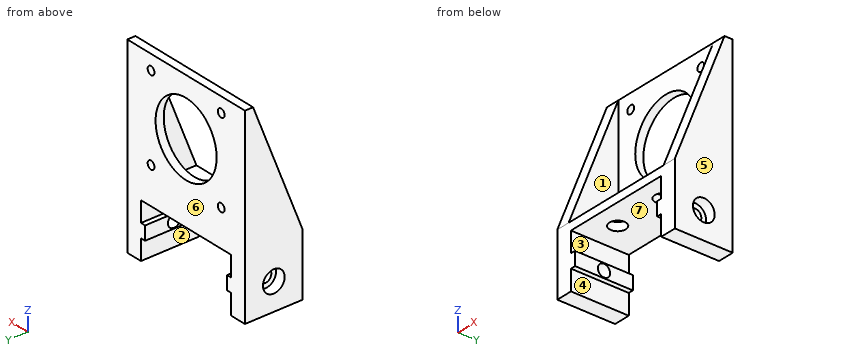
from build123d import *

# Parameters (mm, degrees)
SKETCH1_W           = 42
SKETCH1_H           = 21.3
BOSS_EXTRUDE1_DEPTH = 3
SKETCH2_R           = 3
CUT_EXTRUDE1_DEPTH  = 3
SKETCH4_W           = 42
SKETCH4_H           = 50
SKETCH4_R           = 1.5
SKETCH4_R_2         = 13.5
BOSS_EXTRUDE2_DEPTH = 3
BOSS_EXTRUDE3_DEPTH = 5
BOSS_EXTRUDE4_START = -42
BOSS_EXTRUDE4_DEPTH = 5
SKETCH6_W           = 6.04
SKETCH6_H           = 19.96
BOSS_EXTRUDE5_DEPTH = 21.3
SKETCH8_W           = 1.829995551
SKETCH8_H           = 5.02
BOSS_EXTRUDE6_DEPTH = 21.3
SKETCH7_R           = 2.25
CUT_EXTRUDE2_DEPTH  = 10
SKETCH9_R           = 4
CUT_EXTRUDE3_DEPTH  = 3.8


with BuildPart() as part:
    # Sketch1 → Boss-Extrude1 (new body)
    with BuildSketch(Plane.XY):
        with Locations((98.144783915, 168.215968794)):
            Rectangle(SKETCH1_W, SKETCH1_H)
    extrude(amount=BOSS_EXTRUDE1_DEPTH)

    # Sketch2 → Cut-Extrude1 (cut)
    with BuildSketch(Plane.XY.offset(3)):
        with Locations((108.644783915, 166.065968794)):
            Circle(SKETCH2_R)
        with Locations((88.644783915, 166.065968794)):
            Circle(SKETCH2_R)
    extrude(amount=-CUT_EXTRUDE1_DEPTH, mode=Mode.SUBTRACT)

    # Sketch4 → Boss-Extrude2 (add)
    with BuildSketch(Plane(origin=(0, 178.865968794, 0), x_dir=(-1, 0, 0), z_dir=(0, 1, 0))):
        with Locations((-98.144783915, 25)):
            Rectangle(SKETCH4_W, SKETCH4_H)
        with Locations((-113.644783915, 44.500179206)):
            Circle(SKETCH4_R, mode=Mode.SUBTRACT)
        with Locations((-82.644783915, 44.500179206)):
            Circle(SKETCH4_R, mode=Mode.SUBTRACT)
        with Locations((-82.644783915, 13.500179206)):
            Circle(SKETCH4_R, mode=Mode.SUBTRACT)
        with Locations((-113.644783915, 13.500179206)):
            Circle(SKETCH4_R, mode=Mode.SUBTRACT)
        with Locations((-98.144783915, 29.000179206)):
            Circle(SKETCH4_R_2, mode=Mode.SUBTRACT)
    extrude(amount=-BOSS_EXTRUDE2_DEPTH)

    # Sketch5 → Boss-Extrude3 (add)
    with BuildSketch(Plane(origin=(119.144783915, 0, 0), x_dir=(0, 0, -1), z_dir=(1, 0, 0))):
        Polygon((0, 157.565968794), (0, 178.865968794), (-50, 178.865968794), (-50, 175.865968794), (-3, 157.565968794), align=None)
    extrude(amount=BOSS_EXTRUDE3_DEPTH)

    # Sketch5<3> → Boss-Extrude4 (add)
    with BuildSketch(Plane(origin=(119.144783915, 0, 0), x_dir=(0, 0, -1), z_dir=(1, 0, 0)).offset(BOSS_EXTRUDE4_START)):
        Polygon((0, 157.565968794), (0, 178.865968794), (-50, 178.865968794), (-50, 175.865968794), (-3, 157.565968794), align=None)
    extrude(amount=-BOSS_EXTRUDE4_DEPTH)

    # Sketch6 → Boss-Extrude5 (add)
    with BuildSketch(Plane(origin=(0, 178.865968794, 0), x_dir=(1, 0, 0), z_dir=(0, 1, 0))):
        with Locations((75.164783915, 9.98)):
            Rectangle(SKETCH6_W, SKETCH6_H)
    boss_extrude5 = extrude(amount=-BOSS_EXTRUDE5_DEPTH)

    # Sketch8 → Boss-Extrude6 (add)
    with BuildSketch(Plane(origin=(0, 157.565968794, 0), x_dir=(-1, 0, 0), z_dir=(0, -1, 0))):
        with Locations((-79.099781691, 9.98)):
            Rectangle(SKETCH8_W, SKETCH8_H)
    boss_extrude6 = extrude(amount=-BOSS_EXTRUDE6_DEPTH)

    # Sketch7 → Cut-Extrude2 (cut)
    with BuildSketch(Plane.ZY.offset(-72.144783915)):
        with Locations((-9.98, 168.215968794)):
            Circle(SKETCH7_R)
    cut_extrude2 = extrude(amount=-CUT_EXTRUDE2_DEPTH, mode=Mode.SUBTRACT)

    # Sketch9 → Cut-Extrude3 (cut)
    with BuildSketch(Plane.ZY.offset(-72.144783915)):
        with Locations((-9.98, 168.215968794)):
            Circle(SKETCH9_R)
    cut_extrude3 = extrude(amount=-CUT_EXTRUDE3_DEPTH, mode=Mode.SUBTRACT)

    # Mirror1: Boss-Extrude5, Boss-Extrude6, Cut-Extrude2, Cut-Extrude3 across plane
    add(boss_extrude5.mirror(Plane.ZY.offset(-98.144783915)))
    add(boss_extrude6.mirror(Plane.ZY.offset(-98.144783915)))
    add(cut_extrude2.mirror(Plane.ZY.offset(-98.144783915)), mode=Mode.SUBTRACT)
    add(cut_extrude3.mirror(Plane.ZY.offset(-98.144783915)), mode=Mode.SUBTRACT)


solid = part.part
Can you work these out from the model? Positions are in its coordinate system, mm. Face numbers are marked on the shaded views. A direction names the side the tool comes from. Coordinates: 2 decimals unless noted, no trailing zeros. Loops run counter-clockwise (first coordinate to the right, second up) from the corner with the lowest first, then second, coordinate; pieces in that order, holes last. Notation, with made-up numbers: (24, 25) - (53, 25) arc R15 cw to (53, 32) - close; hole circle Ø7 at (-27, -23). An arc over 180 degrees is marked (long way). Put each result on its own line as item: value. Start each with the question number.
Item 1: Suppose I cut it at B-B (x = 95). Please give me the cut outline in (y, z).
Item 2: Suppose I cut it at D-D (z = -10.5). Please give me the cut outline in (x, y).
Item 3: Which directions (+Z, -Z, +X, -X, +Y, -Y) give clear straight access to the entire face, cutting with the end or side of a thin tool? Please do the marked faces 1, 2 and 3.
Item 4: For pin 1 (5 mm diameter, centred on x = 110, y = 169.5, fed in from -Z); pin 2 (1.5 mm diameter, centred on x = 79, y = 168.5, fed in from +Z); pin 3 (4 mm diameter, centred on x = 113.64, z = 44.5, fed in from -Y), each with a flat end and sliding along its axis, tell me the tip position at first contact or that it passes through.
Item 5: If we mould it in two halves opening along X, with no side actions, what happens to the marked faces 4, 5, 6 and 7? For each: +X half, -X half, draft (parallel to the pull), parting line (faces both ways), or undercut.
Item 6: Suppose I cut it at A-A (z = -3.5). Please give me the cut outline in (x, y).
Item 7: Suppose I cut it at C-C (y = 177.5). Please give me the cut outline in (x, z), and give its area (3 significant figures).
Item 8: If I drill on line 1 along X through (y, z) = (169.5, -4); line 2 along X through (y, z) = (173.75, 17); line 3 along Z through (x, y) = (118, 176.75), over which ranges is the centre line in solid material (lowest first)?
Here are the results:
1. outline: (157.57, 0) - (178.87, 0) - (178.87, 15.87) - (175.87, 15.87) - (175.87, 3) - (157.57, 3) - close; (175.87, 42.13) - (178.87, 42.13) - (178.87, 50) - (175.87, 50) - close
2. outline: (72.14, 157.57) - (80.01, 157.57) - (80.01, 166.03) - (75.94, 166.03) - (75.94, 164.25) - (72.14, 164.25) - close; (72.14, 172.18) - (75.94, 172.18) - (75.94, 170.41) - (80.01, 170.41) - (80.01, 178.87) - (72.14, 178.87) - close; (116.27, 157.57) - (124.14, 157.57) - (124.14, 164.25) - (120.34, 164.25) - (120.34, 166.03) - (116.27, 166.03) - close; (116.27, 170.41) - (120.34, 170.41) - (120.34, 172.18) - (124.14, 172.18) - (124.14, 178.87) - (116.27, 178.87) - close
3. face 1: +Z, -Y
3. face 2: -Z, +Y, -Y
3. face 3: +Y, -Y
4. pin 1: z = 0
4. pin 2: z = 3
4. pin 3: y = 175.87
5. face 4: undercut
5. face 5: +X half
5. face 6: draft
5. face 7: undercut
6. outline: (72.14, 157.57) - (78.18, 157.57) - (78.18, 178.87) - (72.14, 178.87) - close; (118.1, 157.57) - (124.14, 157.57) - (124.14, 178.87) - (118.1, 178.87) - close
7. outline: (72.14, -19.96) - (78.18, -19.96) - (78.18, -12.49) - (80.01, -12.49) - (80.01, -7.47) - (78.18, -7.47) - (78.18, 0) - (118.1, 0) - (118.1, -7.47) - (116.27, -7.47) - (116.27, -12.49) - (118.1, -12.49) - (118.1, -19.96) - (124.14, -19.96) - (124.14, 50) - (72.14, 50) - close; hole circle Ø3 at (82.64, 13.5); hole circle Ø3 at (82.64, 44.5); hole circle Ø27 at (98.14, 29); hole circle Ø3 at (113.64, 13.5); hole circle Ø3 at (113.64, 44.5)
7. area: 2,260 mm²
8. line 1: 72.14 to 78.18, 118.1 to 124.14
8. line 2: 72.14 to 77.14, 119.14 to 124.14
8. line 3: -12.49 to -7.47, 0 to 50
